Geometry check sheet. Reference: the model listing, model coordinates, mm. A direction names the side the tool comes from. Round coordinates to 2 decimals unless told otherwise and drop trailing zeros. Order: outer loops, then holes, each group sorted by start corner. A loop starts at its lowest first (then second) coordinate and runs counter-clockwise, first axis right, second up. Notation, with made-up numbers: (76.5, 84) - (110.5, 84) arc R9 cw to (110.5, 91) - close; hole circle Ø9 at (-6, 3). An arc over 180 degrees is marked (long way). Write each question's results on one line, items separated by ' | '.
```python
from build123d import *

# Parameters (mm, degrees)
SKETCH_2_W          = 69.5
SKETCH_2_H          = 9.9
SKETCH_2_R          = 1.5
SKETCH_2_W_2        = 9.9
SKETCH_2_H_2        = 69.5
EXTRUDE_5_DEPTH     = 2
SKETCH_4_R          = 5
EXTRUDE_8_DEPTH     = 60
SKETCH_6_R          = 3
CUT_EXTRUDE_1_DEPTH = 80.114632022


with BuildPart() as part:
    # 草图2 → 凸台-拉伸5 (new body)
    # profile 1 of 2: a face of its own
    with BuildSketch(Plane(origin=(0, 0, 0), x_dir=(1, 0, 0), z_dir=(0, 1, 0))):
        Rectangle(SKETCH_2_W, SKETCH_2_H)
        with Locations(Location((23.5, 0, 0), (0, 0, 270))):
            Circle(SKETCH_2_R, mode=Mode.SUBTRACT)
        with Locations(Location((10, 0, 0), (0, 0, 270))):
            Circle(SKETCH_2_R, mode=Mode.SUBTRACT)
        with Locations(Location((-23.5, 0, 0), (0, 0, 270))):
            Circle(SKETCH_2_R, mode=Mode.SUBTRACT)
        with Locations(Location((-10, 0, 0), (0, 0, 270))):
            Circle(SKETCH_2_R, mode=Mode.SUBTRACT)
    # profile 2 of 2: a face of its own
    with BuildSketch(Plane(origin=(0, 0, 0), x_dir=(1, 0, 0), z_dir=(0, 1, 0))):
        Rectangle(SKETCH_2_W_2, SKETCH_2_H_2)
        with Locations(Location((0, 10, 0), (0, 0, 270))):
            Circle(SKETCH_2_R, mode=Mode.SUBTRACT)
        with Locations(Location((0, 23.5, 0), (0, 0, 270))):
            Circle(SKETCH_2_R, mode=Mode.SUBTRACT)
        with Locations(Location((0, -23.5, 0), (0, 0, 270))):
            Circle(SKETCH_2_R, mode=Mode.SUBTRACT)
        with Locations(Location((0, -10, 0), (0, 0, 270))):
            Circle(SKETCH_2_R, mode=Mode.SUBTRACT)
    extrude(amount=EXTRUDE_5_DEPTH)

    # 草图4 → 凸台-拉伸8 (add)
    with BuildSketch(Plane(origin=(0, 2, 0), x_dir=(1, 0, 0), z_dir=(0, 1, 0))):
        with Locations(Location((0, 0, 0), (0, 0, 270))):
            Circle(SKETCH_4_R)
    extrude(amount=EXTRUDE_8_DEPTH)

    # 草图6 → 切除-拉伸1 (cut, through all)
    with BuildSketch(Plane.XZ):
        with Locations(Location((0, -30, 0), (0, 0, 270))):
            Circle(SKETCH_6_R)
        with Locations(Location((-30, 0, 0), (0, 0, 270))):
            Circle(SKETCH_6_R)
        with Locations(Location((0, 30, 0), (0, 0, 270))):
            Circle(SKETCH_6_R)
        with Locations(Location((30, 0, 0), (0, 0, 270))):
            Circle(SKETCH_6_R)
    extrude(amount=-CUT_EXTRUDE_1_DEPTH, mode=Mode.SUBTRACT)


solid = part.part
```
(1) Section check D-D (z = 18). Record the cut outline in (x, y).
Answers follow:
outline: (-4.95, 0) - (4.95, 0) - (4.95, 2) - (-4.95, 2) - close
(2) Section check A-A (x = 30). Record the cut outline in (y, z).
Answers follow:
outline: (0, -4.95) - (2, -4.95) - (2, -3) - (0, -3) - close; (0, 3) - (2, 3) - (2, 4.95) - (0, 4.95) - close
(3) Access from +Z, -Z, +X, -X, +Y, -Y to the whole of each face (thin tool, end or side, straight path). Record for faces 1 (the face through (20, 1, 4.95)), 2 (the face through (20, 1, -4.95)), 3 (the face through (-4.95, 1, -20)).
Answers follow:
face 1: +Z, +X, +Y, -Y | face 2: -Z, +X, +Y, -Y | face 3: -Z, -X, +Y, -Y
(4) Material ranges on line 1 (X direction, y = 1.1, z = -30); line 2 (Y direction, x = 1, z = 8); line 3 (X direction, y = 1, z = 23), recorded low to high.
Answers follow:
line 1: -4.95 to -3, 3 to 4.95 | line 2: 0 to 2 | line 3: -4.95 to -1.41, 1.41 to 4.95
(5) Draft check along Z on faces 4 (the face through (0, 1, 33)), 5 (the face through (0.07, 0.99, -11.5)), 6 (the face through (-4.88, 31.58, -1.08)), 7 (the face through (4.95, 1, 20)). Enter one of: released by +Z, released by -Z, zero draft, split by the parting line, or undercut.
Answers follow:
face 4: undercut | face 5: undercut | face 6: split by the parting line | face 7: zero draft
(6) Depth check by flat-ended pin: pin 1 Ø2.5 at (x, z) = (-10, 0) entering from +Y; pin 2 Ø1.6 at (x, y) = (-17.5, 1) entering from -Z; pin 3 Ø4 at (x, z) = (0, 23.5) entering from +Y; pin 4 Ø2 at (y, z) = (1.5, -14) entering from +X. Enter the tip coordinate at first touch or a pass-through.
Answers follow:
pin 1: through | pin 2: z = -4.95 | pin 3: y = 2 | pin 4: x = 4.95
(7) Section check C-C (x = 0). Give the number of separate pieces and of enclosed holes in the cut face, then the cut area to 3 significant figures.
Answers follow:
separate pieces: 7 | enclosed holes: 0 | area: 691 mm²
(8) Section check B-B (z = -23.5). Record the cut outline in (x, y), then the cut area to 3 significant figures.
Answers follow:
outline: (-4.95, 0) - (-1.5, 0) - (-1.5, 2) - (-4.95, 2) - close; (1.5, 0) - (4.95, 0) - (4.95, 2) - (1.5, 2) - close | area: 13.8 mm²
